from build123d import *

# Parameters (mm, degrees)
F0_R     = 12.7
F1_DEPTH = 12.7
F2_DEPTH = 304.8
F3_R     = 5.08
F4_R     = 5.08
F5_R     = 5.08


with BuildPart() as f1:
    # F0 (on Front) → F1 (new body)
    with BuildSketch(Plane.XZ):
        Polygon((76.2, -57.15991), (0, 74.822362), (-76.2, -57.15991), align=None)
        Circle(F0_R, mode=Mode.SUBTRACT)
    extrude(amount=F1_DEPTH)

    # F0 (on Front) → F2 (join)
    with BuildSketch(Plane.XZ):
        Circle(F0_R)
    extrude(amount=F2_DEPTH)

    # F3
    f3_edges = [f1.edges().sort_by_distance(p)[0] for p in [
        (-12.7, -304.8, 0),
    ]]
    fillet(f3_edges, radius=F3_R)

    # F4
    f4_edges = [f1.edges().sort_by_distance(p)[0] for p in [
        (0, -12.7, -57.15991),
    ]]
    fillet(f4_edges, radius=F4_R)

    # F5
    f5_edges = [f1.edges().sort_by_distance(p)[0] for p in [
        (0, 0, -57.15991),
    ]]
    fillet(f5_edges, radius=F5_R)


solid = f1.part
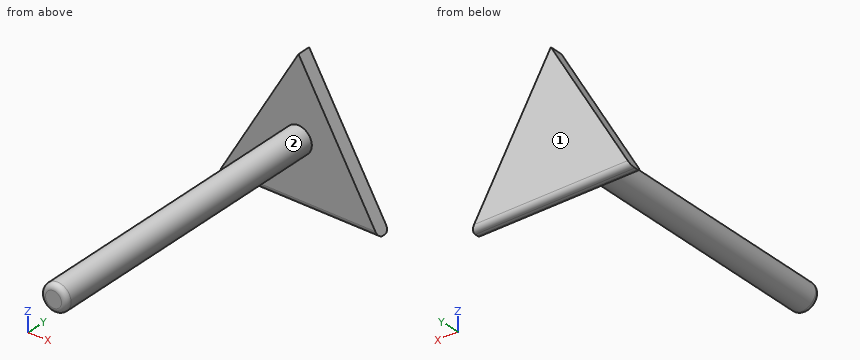
Read the model definition and answer for the solid it produces. Units are mm, in the model's axes. Face numbers are marked on the shaded views. Round coordinates to 2 decimals unless told otherwise and drop trailing zeros. Write each loop counter-clockwise with the first axis right and the second up, starting at its lowest first coordinate (ties: lowest second). Pieces come first, ordered by that corner, then holes.
1. The part is cut by section C-C, the plane x = -49.5. Determine the outline of the cut face in (y, z).
2. Given pin 1 Ø8 at (y, z) = (-166.5, 10.5) entering from -X; pin 2 Ø10 at (x, z) = (-21.5, -11) entering from -Y; pin 3 Ø1.5 at (y, z) = (-94.5, 7.5) entering from -X, each flat-ended and moving along its own axis, determine where each tip first touches the part or whether it passes through.
3. The part is cut by section A-A, the plane z = 0. Determine the outline of the cut face in (x, y).
4. Determine the mould class of the marked faces 1 and 2 for opening direction Z: pulls with the +Z half, pulls with the -Z half, needs draft (parallel to the pull), parting line crosses it, or undercut.
5. Straight lines are drawn through the part: L1, parallel to Y at x = 13, z = 39.5; L2, parallel to Z at x = 1, y = -217; L3, parallel to X at y = -51, z = 10.5. For each, find the intervals that lie inside material, in ascending order.
6. The part is cut by section D-D, the plane z = -37. Determine the outline of the cut face in (x, y), then the cut area to 3 significant figures.
7. The part is cut by section B-B, the plane y = -178.5. Determine the outline of the cut face in (x, z), then the cut area to 3 significant figures.
Values:
1. outline: (-12.7, -52.08) arc R5.08 ccw to (-7.62, -57.16) - (-5.08, -57.16) arc R5.08 ccw to (0, -52.08) - (0, -10.91) - (-12.7, -10.91) - close
2. pin 1: stops at x = -10.91
2. pin 2: stops at y = -12.7
2. pin 3: stops at x = -10.76
3. outline: (-43.2, -12.7) - (-12.7, -12.7) - (-12.7, -299.72) arc R5.08 ccw to (-7.62, -304.8) - (7.62, -304.8) arc R5.08 ccw to (12.7, -299.72) - (12.7, -12.7) - (43.2, -12.7) - (43.2, 0) - (-43.2, 0) - close
4. face 1: needs draft
4. face 2: parting line crosses it
5. L1: y = -12.7 to 0
5. L2: z = -12.66 to 12.66
5. L3: x = -7.14 to 7.14
6. outline: (-64.56, -12.7) - (64.56, -12.7) - (64.56, 0) - (-64.56, 0) - close
6. area: 1,640 mm2
7. outline: circle Ø25.4 at (0, 0)
7. area: 507 mm2
